Can you work these out from the drawing? Everything is in mm from the part's minimum corner. A direction names the side the tool comes from. Round coordinates to 2 decimals unless told otherwise and drop trailing zeros. Write each loop counter-clockwise with the first axis right and the second up, starting at its lowest first coordinate (ties: lowest second). Pieces come first, ordered by that corner, then holes. Notation, with made-up numbers: (-20, 69) -> (34, 69) arc R15 cw to (34, 90) -> close; hole circle Ø5 at (5.25, -28.75). An arc over 180 degrees is marked (long way). One line per question, with ' | ' between items. Start each with the question number.
1. Imagine slicing it at A-A, the plane x = 48. List the corners of the cut face in (y, z) for me.
2. If I drill on line 1 along X through (y, z) = (0.8, 7); line 2 along X through (y, z) = (2.4, 22); line 3 along Z through (x, y) = (68, 3.5), over which ranges is the centre line in solid material (lowest first)? Write a range as [from, to].
3. Imagine slicing it at B-B, the plane z = 11.75. List the corners of the cut face in (x, y) for me, and give its area (3 significant figures).
4. Imagine slicing it at C-C, the plane x = 69. List the corners of the cut face in (y, z) for me.
5. For the marked faces 1 and 2, which set-ups out of +Z, -Z, +X, -X, +Y, -Y let a thin tool reach every point of the face, with its end or its side?
6. For pin 1 Ø2 at (x, z) = (29.5, 23) entering from +Y; pin 2 Ø15.5 at (x, z) = (9.5, 7) entering from +Y; pin 3 Ø0.8 at (x, y) = (28.5, 0.5) entering from -Z; pin 4 Ø5 at (x, z) = (51, 13) entering from -Y, each with a flat end and sliding along its axis, tell me the tip position at first contact or that it passes through.
7. Imagine slicing it at D-D, the plane z = 3.5. List the corners of the cut face in (x, y) for me.
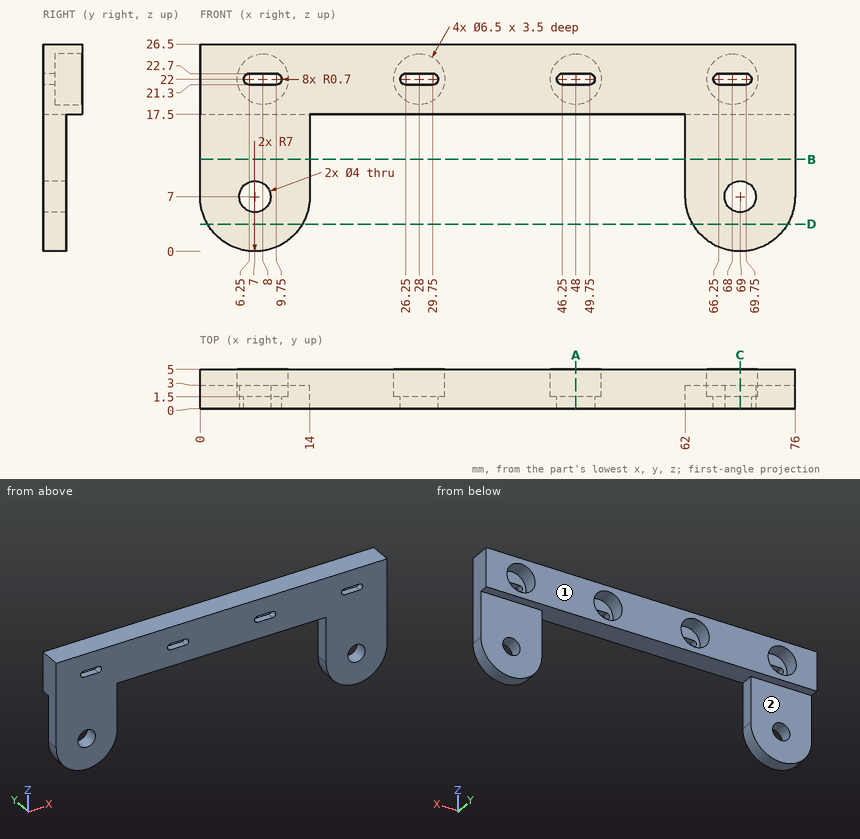
Geometry results:
1) outline: (0, 17.5) -> (5, 17.5) -> (5, 18.75) -> (1.5, 18.75) -> (1.5, 21.3) -> (0, 21.3) -> close; (0, 22.7) -> (1.5, 22.7) -> (1.5, 25.25) -> (5, 25.25) -> (5, 26.5) -> (0, 26.5) -> close
2) line 1: x = [0, 5], [9, 14], [62, 67], [71, 76] | line 2: x = [0, 4.75], [11.25, 24.75], [31.25, 44.75], [51.25, 64.75], [71.25, 76] | line 3: z = [17.5, 18.75], [25.25, 26.5]
3) outline: (0, 0) -> (14, 0) -> (14, 3) -> (0, 3) -> close; (62, 0) -> (76, 0) -> (76, 3) -> (62, 3) -> close | area: 84.0 mm2
4) outline: (0, 0) -> (3, 0) -> (3, 5) -> (0, 5) -> close; (0, 9) -> (3, 9) -> (3, 17.5) -> (5, 17.5) -> (5, 18.91) -> (1.5, 18.91) -> (1.5, 21.3) -> (0, 21.3) -> close; (0, 22.7) -> (1.5, 22.7) -> (1.5, 25.09) -> (5, 25.09) -> (5, 26.5) -> (0, 26.5) -> close
5) face 1: +Z, -Z, +X, -X, +Y | face 2: -Z, +X, -X, +Y
6) pin 1: stops at y = 1.5 | pin 2: stops at y = 3 | pin 3: stops at z = 17.5 | pin 4: passes through
7) outline: (0.94, 0) -> (13.06, 0) -> (13.06, 3) -> (0.94, 3) -> close; (62.94, 0) -> (75.06, 0) -> (75.06, 3) -> (62.94, 3) -> close
